```python
from build123d import *

# Parameters (mm, degrees)
SKETCH1_W           = 50.8
SKETCH1_H           = 38.1
SKETCH1_R           = 2.032
BOSS_EXTRUDE1_DEPTH = 1.27
FILLET3_R           = 2.54
SKETCH2_R           = 2.159
BOSS_EXTRUDE2_DEPTH = 1.27
FILLET6_R           = 2.54


with BuildPart() as part:
    # Sketch1 → Boss-Extrude1 (new body)
    with BuildSketch(Plane.XY):
        Rectangle(SKETCH1_W, SKETCH1_H)
        with Locations((-12.7, 12.7)):
            Circle(SKETCH1_R, mode=Mode.SUBTRACT)
        with Locations((0, 12.7)):
            Circle(SKETCH1_R, mode=Mode.SUBTRACT)
        with Locations((12.7, 12.7)):
            Circle(SKETCH1_R, mode=Mode.SUBTRACT)
        Circle(SKETCH1_R, mode=Mode.SUBTRACT)
        with Locations((12.7, 0)):
            Circle(SKETCH1_R, mode=Mode.SUBTRACT)
        with Locations((0, -12.7)):
            Circle(SKETCH1_R, mode=Mode.SUBTRACT)
        with Locations((12.7, -12.7)):
            Circle(SKETCH1_R, mode=Mode.SUBTRACT)
        with Locations((-12.7, 0)):
            Circle(SKETCH1_R, mode=Mode.SUBTRACT)
        with Locations((-12.7, -12.7)):
            Circle(SKETCH1_R, mode=Mode.SUBTRACT)
    extrude(amount=BOSS_EXTRUDE1_DEPTH)

    # Fillet3
    fillet3_edges = [part.edges().sort_by_distance(p)[0] for p in [
        (25.4, -19.05, 0.635),
        (25.4, 19.05, 0.635),
    ]]
    fillet(fillet3_edges, radius=FILLET3_R)

    # Sketch2 → Boss-Extrude2 (add)
    with BuildSketch(Plane.XY.offset(1.27)):
        Polygon((-25.4, -25.4), (-25.4, -19.05), (-25.4, 19.05), (-25.4, 25.4), (-48.641, 25.4), (-48.641, -25.4), align=None)
        with Locations((-42.291, -19.05)):
            Circle(SKETCH2_R, mode=Mode.SUBTRACT)
        with Locations((-42.291, 0)):
            Circle(SKETCH2_R, mode=Mode.SUBTRACT)
        with Locations((-42.291, 19.05)):
            Circle(SKETCH2_R, mode=Mode.SUBTRACT)
    extrude(amount=-BOSS_EXTRUDE2_DEPTH)

    # Fillet6
    fillet6_edges = [part.edges().sort_by_distance(p)[0] for p in [
        (-25.4, 25.4, 0.635),
        (-25.4, -25.4, 0.635),
        (-48.641, -25.4, 0.635),
        (-48.641, 25.4, 0.635),
        (-25.4, -19.05, 0.635),
        (-25.4, 19.05, 0.635),
    ]]
    fillet(fillet6_edges, radius=FILLET6_R)


solid = part.part
```
Could you check a few things on this model? Use its own coordinates, in mm. Round coordinates to 2 decimals unless told otherwise and drop trailing zeros. Loops run counter-clockwise (first coordinate to the right, second up) from the corner with the lowest first, then second, coordinate; pieces in that order, holes last.
Q1. I want a section at B-B (x = -41). Write out the boundary of the cut face in (y, z), and give its area (3 significant figures).
Q2. Thinking about a two-plate mould opening in X: for faces 1 (the flat face through (-20, 0, 1.27)), 2 (the cylindrical face through (-44.45, 0.09, 0.64)), 3 (the cylindrical face through (-24.676, 19.814, 0.644)), which applies, pulls with the +X half, pulls with the -X half, needs draft (parallel to the pull), parting line crosses it, or undercut?
Q3. Please list where these lines run through material, in increasing order: L1, parallel to Y at x = 12.7, z = 1.05; L2, parallel to X at y = -0.5, z = 0.8.
Q4. For P1, Ø3.5, axis at x = 12.7, y = 0, coming from the -Z side, with a flat end and sliding along its axis, tell me the tip position at first contact or that it passes through.
Q5. I want a section at A-A (y = -12.7). Write out the boundary of the cut face in (x, z).
Q6. I want a section at C-C (z = 0.9). Give the number of separate pieces and of enclosed holes in the cut face, and give its area (3 significant figures).
Q7. I want a section at D-D (x = 6). Write out the boundary of the cut face in (y, z).
Answer below:
1. outline: (-25.4, 0) - (-20.78, 0) - (-20.78, 1.27) - (-25.4, 1.27) - close; (-17.32, 0) - (-1.73, 0) - (-1.73, 1.27) - (-17.32, 1.27) - close; (1.73, 0) - (17.32, 0) - (17.32, 1.27) - (1.73, 1.27) - close; (20.78, 0) - (25.4, 0) - (25.4, 1.27) - (20.78, 1.27) - close
1. area: 51.3 mm2
2. face 1: needs draft
2. face 2: undercut
2. face 3: pulls with the +X half
3. L1: y = -19.05 to -14.73, -10.67 to -2.03, 2.03 to 10.67, 14.73 to 19.05
3. L2: x = -48.64 to -44.39, -40.19 to -14.67, -10.73 to -1.97, 1.97 to 10.73, 14.67 to 25.4
4. P1: passes through
5. outline: (-48.64, 0) - (-14.73, 0) - (-14.73, 1.27) - (-48.64, 1.27) - close; (-10.67, 0) - (-2.03, 0) - (-2.03, 1.27) - (-10.67, 1.27) - close; (2.03, 0) - (10.67, 0) - (10.67, 1.27) - (2.03, 1.27) - close; (14.73, 0) - (25.4, 0) - (25.4, 1.27) - (14.73, 1.27) - close
6. separate pieces: 1
6. enclosed holes: 12
6. area: 2,950 mm2
7. outline: (-19.05, 0) - (19.05, 0) - (19.05, 1.27) - (-19.05, 1.27) - close
